The model under review builds one solid part; all positions refer to its coordinate system, in mm. A direction names the side the tool comes from. Round coordinates to 2 decimals unless told otherwise and drop trailing zeros. Loops run counter-clockwise (first coordinate to the right, second up) from the corner with the lowest first, then second, coordinate; pieces in that order, holes last. Notation, with made-up numbers: (-31, 86) - (-2, 86) arc R22 ccw to (-2, 117) - close; hole circle Ø2 at (87, -37). An arc over 180 degrees is marked (long way). Answer as CSV lines item,"result".
from build123d import *

# Parameters (mm, degrees)
SKETCH1_R           = 2.5
BOSS_EXTRUDE1_DEPTH = 3


with BuildPart() as part:
    # Sketch1 → Boss-Extrude1 (new body)
    with BuildSketch(Plane.XY):
        with BuildLine():
            Line((167.77621964, -174.96032759), (287.77621964, -174.96032759))
            ThreePointArc((287.77621964, -174.96032759), (308.989423075, -166.173531026), (317.77621964, -144.96032759))
            Line((317.77621964, -144.96032759), (317.77621964, -92.46032759))
            ThreePointArc((317.77621964, -92.46032759), (325.27621964, -84.96032759), (317.77621964, -77.46032759))
            Line((317.77621964, -77.46032759), (317.77621964, -24.96032759))
            ThreePointArc((317.77621964, -24.96032759), (308.989423075, -3.747124154), (287.77621964, 5.03967241))
            Line((287.77621964, 5.03967241), (167.77621964, 5.03967241))
            ThreePointArc((167.77621964, 5.03967241), (146.563016204, -3.747124154), (137.77621964, -24.96032759))
            Line((137.77621964, -24.96032759), (137.77621964, -77.46032759))
            ThreePointArc((137.77621964, -77.46032759), (130.27621964, -84.96032759), (137.77621964, -92.46032759))
            Line((137.77621964, -92.46032759), (137.77621964, -144.96032759))
            ThreePointArc((137.77621964, -144.96032759), (146.563016204, -166.173531026), (167.77621964, -174.96032759))
        make_face()
        with Locations((317.77621964, -84.96032759)):
            Circle(SKETCH1_R, mode=Mode.SUBTRACT)
        with Locations((137.77621964, -84.96032759)):
            Circle(SKETCH1_R, mode=Mode.SUBTRACT)
        with BuildLine():
            Line((226.284678956, -14.96032759), (167.784678956, -14.96032759))
            ThreePointArc((167.784678956, -14.96032759), (160.713611144, -17.889259778), (157.784678956, -24.96032759))
            Line((157.784678956, -24.96032759), (150.784678956, -24.96032759))
            Line((150.784678956, -24.96032759), (150.784678956, -74.96032759))
            Line((150.784678956, -74.96032759), (157.784678956, -74.96032759))
            Line((157.784678956, -74.96032759), (157.784678956, -83.46032759))
            Line((157.784678956, -83.46032759), (147.784678956, -83.46032759))
            Line((147.784678956, -83.46032759), (147.784678956, -86.46032759))
            Line((147.784678956, -86.46032759), (157.784678956, -86.46032759))
            Line((157.784678956, -86.46032759), (157.77621964, -92.46032759))
            Line((157.77621964, -92.46032759), (157.77621964, -106.96032759))
            ThreePointArc((157.77621964, -106.96032759), (160.705151828, -114.031395402), (167.77621964, -116.96032759))
            Line((167.77621964, -116.96032759), (182.77621964, -116.96032759))
            Line((182.77621964, -116.96032759), (182.77621964, -131.96032759))
            Line((182.77621964, -131.96032759), (157.77621964, -131.96032759))
            Line((157.77621964, -131.96032759), (157.77621964, -134.96032759))
            Line((157.77621964, -134.96032759), (297.77621964, -134.96032759))
            Line((297.77621964, -134.96032759), (297.77621964, -131.96032759))
            Line((297.77621964, -131.96032759), (272.77621964, -131.96032759))
            Line((272.77621964, -131.96032759), (272.77621964, -116.96032759))
            Line((272.77621964, -116.96032759), (287.77621964, -116.96032759))
            ThreePointArc((287.77621964, -116.96032759), (294.847287452, -114.031395402), (297.77621964, -106.96032759))
            Line((297.77621964, -106.96032759), (297.77621964, -92.46032759))
            Line((297.77621964, -92.46032759), (297.784678956, -86.46032759))
            Line((297.784678956, -86.46032759), (307.784678956, -86.46032759))
            Line((307.784678956, -86.46032759), (307.784678956, -83.46032759))
            Line((307.784678956, -83.46032759), (297.784678956, -83.46032759))
            Line((297.784678956, -83.46032759), (297.784678956, -74.96032759))
            Line((297.784678956, -74.96032759), (304.784678956, -74.96032759))
            Line((304.784678956, -74.96032759), (304.784678956, -24.96032759))
            Line((304.784678956, -24.96032759), (297.784678956, -24.96032759))
            ThreePointArc((297.784678956, -24.96032759), (294.855746768, -17.889259778), (287.784678956, -14.96032759))
            Line((287.784678956, -14.96032759), (229.284678956, -14.96032759))
            Line((229.284678956, -14.96032759), (226.284678956, -14.96032759))
        make_face(mode=Mode.SUBTRACT)
    extrude(amount=BOSS_EXTRUDE1_DEPTH)


solid = part.part
1. Draft analysis for pull direction Y (two halves, no side actions). For faces 3 (the face through (320.086, -85.918, 1.479)), 4 (the face through (325.274, -85.125, 1.479)), 5 (the face through (226, -144, 3)), state which applies: +Y half, -Y half, draft (parallel to the pull), parting line (faces both ways), or undercut.
Numbers:
face 3,"undercut"
face 4,"parting line"
face 5,"draft"
2. Take a section at B-B (x = 228). State the section outline as (y, z) points, plus the area to 3 significant figures.
Numbers:
outline,"(-174.96, 0) - (-134.96, 0) - (-134.96, 3) - (-174.96, 3) - close; (-14.96, 0) - (5.04, 0) - (5.04, 3) - (-14.96, 3) - close"
area,"180 mm²"
3. Take a section at A-A (y = -28). State the section outline as (x, z) points, plus the area to 3 significant figures.
Numbers:
outline,"(137.78, 0) - (150.78, 0) - (150.78, 3) - (137.78, 3) - close; (304.78, 0) - (317.78, 0) - (317.78, 3) - (304.78, 3) - close"
area,"78.0 mm²"
4. Clearance check with flat-ended pins moving along their axes: pin 1 (1.5 mm diameter, centred on x = 155.5, z = 1, fed in from -Y); pin 2 (1.5 mm diameter, centred on y = -44, z = 1, fed in from -X); pin 3 (8 mm diameter, centred on x = 163.5, y = -30.5, fed in from -Z); pin 4 (0.9 mm diameter, centred on x = 153.5, z = 1.5, fed in from -Y). State where each tip first meets the part, or that it passes through.
Numbers:
pin 1,"stops at y = -172.66"
pin 2,"stops at x = 137.78"
pin 3,"passes through"
pin 4,"stops at y = -171.58"
5. Take a section at D-D (y = -153). State the section outline as (x, z) points, plus the area to 3 significant figures.
Numbers:
outline,"(138.87, 0) - (316.68, 0) - (316.68, 3) - (138.87, 3) - close"
area,"533 mm²"
6. Take a section at C-C (z = 1.1). State how many separate pieces and enclosed holes the cut face has, plus the area to 3 significant figures.
Numbers:
separate pieces,"1"
enclosed holes,"3"
area,"15,000 mm²"
7. Tool access review of faces 1 (the face through (160.628, -113.953, 1.479)), 2 (the face through (130.278, -84.795, 1.479)): name each direction out of +Z, -Z, +X, -X, +Y, -Y from which nothing blocks a thin tool from reaching the whole face with its end or side.
Numbers:
face 1,"+Z, -Z"
face 2,"+Z, -Z, -X"
8. Wall thickness on probe 1 along Y at (x, z) = (174.5, 0.7); probe 2 along Y at (x, z) = (262.5, 0.6); probe 3 along X at (y, z) = (-130, 2.6): over which ranges is each line inside the solid? List them lowest first.
Numbers:
probe 1,"y = -174.96 to -134.96, -131.96 to -116.96, -14.96 to 5.04"
probe 2,"y = -174.96 to -134.96, -14.96 to 5.04"
probe 3,"x = 137.78 to 182.78, 272.78 to 317.78"
